```python
from build123d import *

# Parameters (mm, degrees)
F0_R     = 6.35
F1_DEPTH = 10
F0_R_2   = 19.05
F2_DEPTH = 44
F3_DEPTH = 38
F4_R     = 6.6505969319
F5_DEPTH = 14.8986119061


with BuildPart() as f1:
    # F0 (on Top) → F1 (new body)
    with BuildSketch(Plane.XY):
        with BuildLine():
            Line((63.5, 31.75), (-63.5, 31.75))
            Line((-63.5, 31.75), (-63.5, -31.75))
            Line((-63.5, -31.75), (-12.7, -31.75))
            Line((-12.7, -31.75), (-12.7, -21.9970452561))
            ThreePointArc((-12.7, -21.9970452561), (-12.7, 21.9970452561), (25.4, 0))
            ThreePointArc((25.4, 0), (21.9970452561, -12.7), (12.7, -21.9970452561))
            Line((12.7, -21.9970452561), (12.7, -31.75))
            Line((12.7, -31.75), (63.5, -31.75))
            Line((63.5, -31.75), (63.5, 31.75))
        make_face()
        with Locations((-53.34, -21.59)):
            Circle(F0_R, mode=Mode.SUBTRACT)
        with Locations((53.34, -21.59)):
            Circle(F0_R, mode=Mode.SUBTRACT)
        with Locations((-53.34, 21.59)):
            Circle(F0_R, mode=Mode.SUBTRACT)
        with Locations((53.34, 21.59)):
            Circle(F0_R, mode=Mode.SUBTRACT)
    extrude(amount=F1_DEPTH)

    # F0 (on Top) → F2 (join)
    with BuildSketch(Plane.XY):
        with BuildLine():
            ThreePointArc((25.4, 0), (-12.7, 21.9970452561), (-12.7, -21.9970452561))
            ThreePointArc((-12.7, -21.9970452561), (0, -25.4), (12.7, -21.9970452561))
            ThreePointArc((12.7, -21.9970452561), (21.9970452561, -12.7), (25.4, 0))
        make_face()
        Circle(F0_R_2, mode=Mode.SUBTRACT)
    extrude(amount=F2_DEPTH)

    # F0 (on Top) → F3 (join)
    with BuildSketch(Plane.XY):
        with BuildLine():
            Line((-12.7, -21.9970452561), (-12.7, -31.75))
            Line((-12.7, -31.75), (12.7, -31.75))
            Line((12.7, -31.75), (12.7, -21.9970452561))
            ThreePointArc((12.7, -21.9970452561), (0, -25.4), (-12.7, -21.9970452561))
        make_face()
    extrude(amount=F3_DEPTH)

    # F4 (on face) → F5 (cut, up to face)
    with BuildSketch(Plane.XZ.offset(31.75)):
        with Locations((0, 25.4719480872)):
            Circle(F4_R)
    extrude(amount=-F5_DEPTH, mode=Mode.SUBTRACT)


solid = f1.part
```
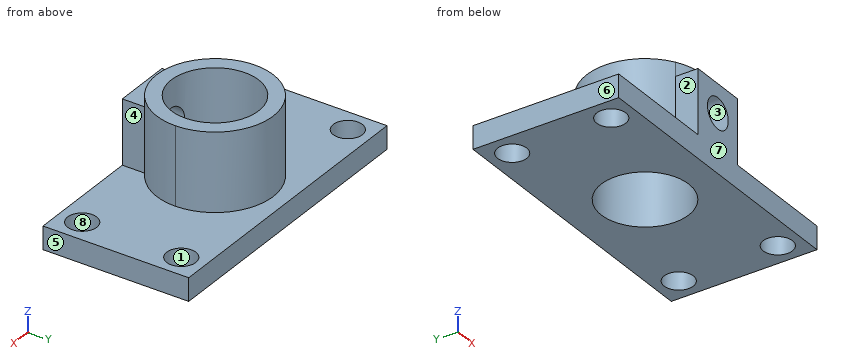
Part model, mm, in its own coordinate system. Face numbers are marked on the shaded views. A direction names the side the tool comes from. Coordinates: 2 decimals unless noted, no trailing zeros. Order: outer loops, then holes, each group sorted by start corner. A loop starts at its lowest first (then second) coordinate and runs counter-clockwise, first axis right, second up. Notation, with made-up numbers: (-37, -21.5) - (22, -21.5) arc R31 cw to (22, 17.5) - close; hole circle Ø1 at (-32, -10.5). An arc over 180 degrees is marked (long way). Return JSON: item names as keys, results as strings. Group by question number.
Item 1: Cut at C-C (y = -16.5). List the corners of the cut face in (x, z).
Item 2: Which spindle directions (+Z, -Z, +X, -X, +Y, -Y) get a long thin tool onto all of the face, cutting with end or side? Do the marked faces 1, 2, 3, 4 and 5. Say none if no direction does.
Item 3: Cut at D-D (y = 6.5). List the corners of the cut face in (x, z).
Item 4: Cut at B-B (z = 35). List the corners of the cut face in (x, y).
Item 5: Pin check, flat tips, straight feed: pin 1 (11.5 mm diameter, centred on x = -53.34, y = -21.59, fed in from -Z); pin 2 (1 mm diameter, centred on y = -3.5, z = 33.5, fed in from -X); pin 3 (4 mm diameter, centred on x = 4, z = 36, fed in from +Y); pin 4 (5 mm diameter, centred on x = 46, y = -2.5, fed in from +Z). Stop position of each tip, or through.
Item 6: Pull direction X, two halves, no side cores. Call the marked faces 6, 7 and 8: pulls with the +X half, pulls with the -X half, needs draft (parallel to the pull), parting line crosses it, or undercut.
Item 7: Drill centre lines: probe 1 along X at (y, z) = (-21, 5); probe 2 along Y at (x, z) = (53, 5); probe 3 along X at (y, z) = (-1, 11). Where is each one in solid material? Low to high. Write a range as from..to.
Item 8: Cut at A-A (x = 53.34). List the corners of the cut face in (y, z), plus the area to 3 significant figures.
Check values:
{
 "1": {"outline": "(-63.5, 0) - (-57.14, 0) - (-57.14, 10) - (-63.5, 10) - close; (-49.54, 0) - (-9.52, 0) - (-9.52, 44) - (-19.31, 44) - (-19.31, 10) - (-49.54, 10) - close; (9.52, 0) - (49.54, 0) - (49.54, 10) - (19.31, 10) - (19.31, 44) - (9.52, 44) - close; (57.14, 0) - (63.5, 0) - (63.5, 10) - (57.14, 10) - close"},
 "2": {"face 1": "+Z, -Z", "face 2": "+Z, -X, -Y", "face 3": "-Y", "face 4": "+Z, +X, -Y", "face 5": "+Z, -Z, +X, +Y, -Y"},
 "3": {"outline": "(-63.5, 0) - (-17.91, 0) - (-17.91, 44) - (-24.55, 44) - (-24.55, 10) - (-63.5, 10) - close; (17.91, 0) - (63.5, 0) - (63.5, 10) - (24.55, 10) - (24.55, 44) - (17.91, 44) - close"},
 "4": {"outline": "(-12.7, -31.75) - (12.7, -31.75) - (12.7, -22) arc R25.4 ccw (long way) to (-12.7, -22) - close; hole circle Ø38.1 at (0, 0)"},
 "5": {"pin 1": "passes through", "pin 2": "stops at x = -25.22", "pin 3": "stops at y = 25.32", "pin 4": "stops at z = 10"},
 "6": {"face 6": "pulls with the -X half", "face 7": "needs draft", "face 8": "undercut"},
 "7": {"probe 1": "x = -63.5..-59.66, -47.02..47.02, 59.66..63.5", "probe 2": "y = -31.75..-27.93, -15.25..15.25, 27.93..31.75", "probe 3": "x = -25.38..-19.02, 19.02..25.38"},
 "8": {"outline": "(-31.75, 0) - (-27.94, 0) - (-27.94, 10) - (-31.75, 10) - close; (-15.24, 0) - (15.24, 0) - (15.24, 10) - (-15.24, 10) - close; (27.94, 0) - (31.75, 0) - (31.75, 10) - (27.94, 10) - close", "area": "381 mm2"}
}
